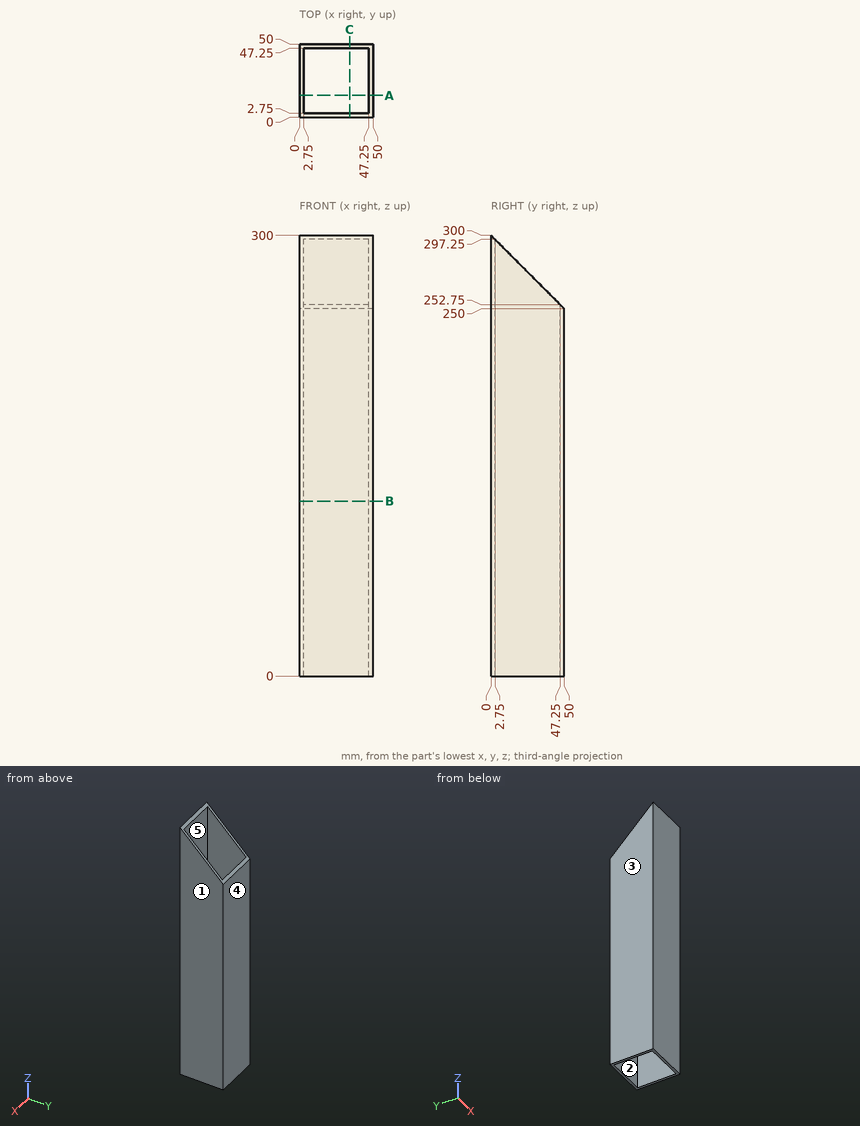
Study the drawing (mm; zero at the part's minimum x, y, z) and answer. A direction names the side the tool comes from. Give positions to 0.01 mm unless a question says otherwise; leave off trailing zeros. Write each loop counter-clockwise with the first axis right and the second up, starting at its lowest first coordinate (ties: lowest second). Pieces come first, ordered by that corner, then holes. Notation, with made-up numbers: (3.5, 82) - (62.5, 82) arc R5 cw to (62.5, 89) - close; hole circle Ø6 at (6.5, 62). An arc over 180 degrees is marked (long way). Write item = value, one per line. Start each with the question number.
Item 1: Find the intervals of material crossed by probe 1 along Y at (x, z) = (9, 71.5); probe 2 along Y at (x, z) = (43.5, 275), in increasing order. Write a range as [from, to].
Item 2: This flat-tipped pin is pushed along its axis until it touches: P1, Ø5, axis at x = 7.5, y = 18, coming from the -Z side. Where does it stop, or does it pass through?
Item 3: Find section B-B (z = 119). Give the vertices of the cut face in (x, y).
Item 4: A tool of negligible diameter and unlimited length cuts with its end or side. For the marked faces 1 and 2, from which of +Z, -Z, +X, -X, +Y, -Y can it reach the whole face along a straight path? Write none if from no direction.
Item 5: Find section A-A (y = 15). Give the vertices of the cut face in (x, z), then the cut area to 3 significant figures.
Item 6: The mould has two halves that part along Y. Classify the marked faces 3, 4 and 5: +Y half, -Y half, draft (parallel to the pull), parting line (faces both ways), or undercut.
Item 7: Find section C-C (x = 34). Give the vertices of the cut face in (y, z), then the cut area to 3 significant figures.
Response:
q1.probe_1 = [0, 2.75], [47.25, 50]
q1.probe_2 = [0, 2.75]
q2.P1 = through
q3.outline = (0, 0) - (50, 0) - (50, 50) - (0, 50) - close; hole (2.75, 2.75) - (47.25, 2.75) - (47.25, 47.25) - (2.75, 47.25) - close
q4.face_1 = +Z, -Z, +X, +Y, -Y
q4.face_2 = +Z, -Z
q5.outline = (0, 0) - (2.75, 0) - (2.75, 285) - (0, 285) - close; (47.25, 0) - (50, 0) - (50, 285) - (47.25, 285) - close
q5.area = 1,570 mm²
q6.face_3 = draft
q6.face_4 = +Y half
q6.face_5 = undercut
q7.outline = (0, 0) - (2.75, 0) - (2.75, 297.25) - (0, 300) - close; (47.25, 0) - (50, 0) - (50, 250) - (47.25, 252.75) - close
q7.area = 1,510 mm²
